Part model, mm, in its own coordinate system. Face numbers are marked on the shaded views. A direction names the side the tool comes from. Round coordinates to 2 decimals unless told otherwise and drop trailing zeros. Write each loop counter-clockwise with the first axis right and the second up, starting at its lowest first coordinate (ties: lowest second). Pieces come first, ordered by that corner, then holes. Notation, with made-up numbers: (44, 84) -> (87, 84) arc R16 cw to (87, 107) -> close; hole circle Ø8 at (67, -27.5). An arc over 180 degrees is marked (long way). Return JSON: item names as keys, results as strings. Group by question number.
(1) Saw through at C-C (y = 143). List the corners of the cut face in (x, z).
(2) Saw through at D-D (y = -368). List the corners of the cut face in (x, z).
(3) Drop flat-ended pins along their axis: pin 1 Ø6 at (y, z) = (-218, 209) entering from -X; pin 2 Ø4 at (x, z) = (337.5, 376.5) entering from -Y; pin 3 Ø6 at (x, y) = (418.5, -172) entering from +Z. Give the stop position or say it passes through.
(4) Drill centre lines: L1, parallel to Y at x = 434, z = 42.5; L2, parallel to Y at x = 382.5, z = 96; L3, parallel to Z at x = 487, y = 117.5. Where is each one in solid material? Low to high. Write a range as from..to.
(5) Mould opens along Z. For the marked faces 1, 2 and 3 say: +Z half, -Z half, draft (parallel to the pull), parting line (faces both ways), or undercut.
(6) Tool access for the marked faces 4, 5, 6 and 7: list every direction of +Z, -Z, +X, -X, +Y, -Y with a clear straight run to the whole face (end or side of a thin tool).
(7) Saw through at B-B (z = 155). State how many separate pieces and enclosed holes the cut face has, plus the area to 3 significant figures.
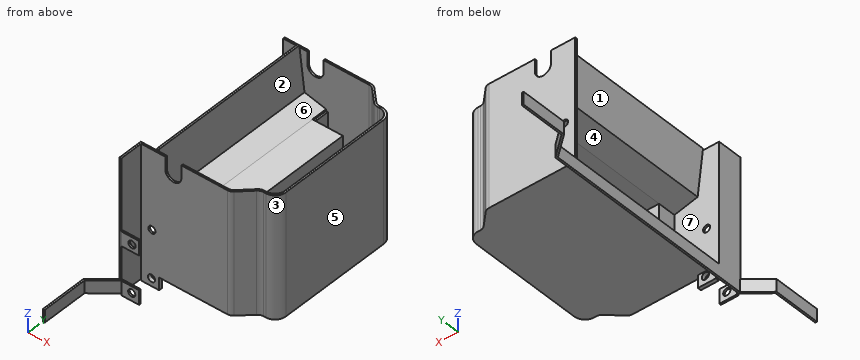
from build123d import *

# Parameters (mm, degrees)
F7_START  = 35
F7_DEPTH  = 5
F8_START  = 5
F8_DEPTH  = 35
F11_DEPTH = 200
F13_DEPTH = 369.76
F15_DEPTH = 45
F17_DEPTH = 45
F18_DEPTH = 45
F19_DEPTH = 45
F20_DEPTH = 335
F22_W     = 50.1510878829
F22_H     = 10
F23_DEPTH = 35
F24_W     = 5
F24_H     = 35
F24_H_2   = 5
F25_DEPTH = 50
F26_R     = 10
F27_DEPTH = 255.001
F29_DEPTH = 335
F30_W     = 5
F30_H     = 40
F31_DEPTH = 50
F32_R     = 10
F33_DEPTH = 780.001
F35_DEPTH = 715.001


with BuildPart() as f7:
    # F5 (on face) → F7 (new body)
    with BuildSketch(Plane.XY.offset(F7_START)):
        with BuildLine():
            Line((536.0502983732, 235), (295.2061215611, 235))
            Line((295.2061215611, 235), (295.2061215611, -235))
            Line((295.2061215611, -235), (536.0502983732, -235))
            ThreePointArc((536.0502983732, -235), (543.6023308733, -233.5193629782), (550.0361814825, -229.2966805117))
            Line((550.0361814825, -229.2966805117), (584.3760616397, -195.7033194883))
            ThreePointArc((584.3760616397, -195.7033194883), (590.8099122489, -191.4806370218), (598.361944749, -190))
            Line((598.361944749, -190), (605.2061215611, -190))
            ThreePointArc((605.2061215611, -190), (626.4193249967, -181.2132034356), (635.2061215611, -160))
            Line((635.2061215611, -160), (635.2061215611, 160))
            ThreePointArc((635.2061215611, 160), (626.4193249967, 181.2132034356), (605.2061215611, 190))
            Line((605.2061215611, 190), (598.361944749, 190))
            ThreePointArc((598.361944749, 190), (590.8099122489, 191.4806370218), (584.3760616397, 195.7033194883))
            Line((584.3760616397, 195.7033194883), (550.0361814825, 229.2966805117))
            ThreePointArc((550.0361814825, 229.2966805117), (543.6023308733, 233.5193629782), (536.0502983732, 235))
        make_face()
    extrude(amount=F7_DEPTH)

    # F10 (on face) → F11 (join)
    with BuildSketch(Plane.XY.offset(40)):
        Polygon((420.2061215611, 230), (415.2061215611, 230), (415.2061215611, 179.7606539726), (495.2061215611, 179.7606539726), (495.2061215611, -180), (415.2061215611, -180), (415.2061215611, -230), (420.2061215611, -230), (420.2061215611, -185), (500.2061215611, -185), (500.2061215611, 184.7606539726), (420.2061215611, 184.7606539726), align=None)
    extrude(amount=F11_DEPTH)



with BuildPart() as f8:
    # F6 (on face) → F8 (new body)
    with BuildSketch(Plane.XY.offset(F8_START)):
        Polygon((235.3396033727, 350), (235.3396033727, 480), (230.3396033727, 480), (230.3396033727, 347.6614641333), (290.2061215611, 297.6614641333), (290.2061215611, -297.6614641333), (230.3396033727, -347.6614641333), (230.3396033727, -480), (235.3396033727, -480), (235.3396033727, -350), (295.2061215611, -300), (295.2061215611, 300), align=None)
    extrude(amount=F8_DEPTH)


with BuildPart() as f13:
    # F12 (on face) → F13 (new body)
    with BuildSketch(Plane.XZ.offset(185)):
        Polygon((415.077149868, 240), (500.2061215611, 240), (500.2061215611, 245), (415.6496353582, 245), (354.7629135856, 259.1279170394), (340.264830222, 380.0120656257), (335.2289983824, 380.0120656257), (350.2161502838, 255.0500929356), align=None)
    extrude(amount=-F13_DEPTH)

    # F14 (on face) → F15 (join)
    with BuildSketch(Plane.XZ.offset(185)):
        Polygon((354.7629135856, 259.1279170394), (350.2161502838, 255.0500929356), (415.077149868, 240), (415.077149868, 245.1328372965), align=None)
    extrude(amount=F15_DEPTH)

    # F16 (on face) → F17 (join)
    with BuildSketch(Plane(origin=(0, 184.76, 0), x_dir=(-1, 0, 0), z_dir=(0, 1, 0))):
        Polygon((-415.077149868, 245.1328372965), (-415.077149868, 240), (-350.2161502838, 255.0500929356), (-354.7629135856, 259.1279170394), align=None)
    extrude(amount=F17_DEPTH)

    # F18 (add): a face of the model
    f18_faces = [f13.faces().sort_by_distance(p)[0] for p in [
        (345.1049776592, -185, 318.5448987695),
    ]]
    extrude(f18_faces, amount=F18_DEPTH)

    # F19 (add): a face of the model
    f19_faces = [f13.faces().sort_by_distance(p)[0] for p in [
        (345.1049776592, 184.76, 318.5448987695),
    ]]
    extrude(f19_faces, amount=F19_DEPTH)


with BuildPart() as f7_1:
    add(f7.part)

    add(f8.part)  # F20 merges F8

    add(f13.part)  # F20 merges F13
    # F9 (on face) → F20 (join)
    with BuildSketch(Plane.XY.offset(40)):
        with BuildLine():
            Line((536.0502983732, 235), (295.2061215611, 235))
            Line((295.2061215611, 235), (295.2061215611, 230))
            Line((295.2061215611, 230), (534.0113425762, 230))
            ThreePointArc((534.0113425762, 230), (541.5633750764, 228.5193629782), (547.9972256855, 224.2966805117))
            Line((547.9972256855, 224.2966805117), (582.3371058428, 190.7033194883))
            ThreePointArc((582.3371058428, 190.7033194883), (588.7709564519, 186.4806370218), (596.322988952, 185))
            Line((596.322988952, 185), (602.2061215611, 185))
            ThreePointArc((602.2061215611, 185), (622.0051114343, 176.7989898732), (630.2061215611, 157))
            Line((630.2061215611, 157), (630.2061215611, -157))
            ThreePointArc((630.2061215611, -157), (622.0051114343, -176.7989898732), (602.2061215611, -185))
            Line((602.2061215611, -185), (596.322988952, -185))
            ThreePointArc((596.322988952, -185), (588.7709564519, -186.4806370218), (582.3371058428, -190.7033194883))
            Line((582.3371058428, -190.7033194883), (547.9972256855, -224.2966805117))
            ThreePointArc((547.9972256855, -224.2966805117), (541.5633750764, -228.5193629782), (534.0113425762, -230))
            Line((534.0113425762, -230), (295.2061215611, -230))
            Line((295.2061215611, -230), (295.2061215611, -235))
            Line((295.2061215611, -235), (536.0502983732, -235))
            ThreePointArc((536.0502983732, -235), (543.6023308733, -233.5193629782), (550.0361814825, -229.2966805117))
            Line((550.0361814825, -229.2966805117), (584.3760616397, -195.7033194883))
            ThreePointArc((584.3760616397, -195.7033194883), (590.8099122489, -191.4806370218), (598.361944749, -190))
            Line((598.361944749, -190), (605.2061215611, -190))
            ThreePointArc((605.2061215611, -190), (626.4193249967, -181.2132034356), (635.2061215611, -160))
            Line((635.2061215611, -160), (635.2061215611, 160))
            ThreePointArc((635.2061215611, 160), (626.4193249967, 181.2132034356), (605.2061215611, 190))
            Line((605.2061215611, 190), (598.361944749, 190))
            ThreePointArc((598.361944749, 190), (590.8099122489, 191.4806370218), (584.3760616397, 195.7033194883))
            Line((584.3760616397, 195.7033194883), (550.0361814825, 229.2966805117))
            ThreePointArc((550.0361814825, 229.2966805117), (543.6023308733, 233.5193629782), (536.0502983732, 235))
        make_face()
    extrude(amount=F20_DEPTH)

    # F22 (on face) → F23 (join)
    with BuildSketch(Plane(origin=(0, 0, 35), x_dir=(1, 0, 0), z_dir=(0, 0, -1))):
        with Locations((320.2816655026, 230)):
            Rectangle(F22_W, F22_H)
    extrude(amount=F23_DEPTH)

    # F24 (on face) → F25 (join)
    with BuildSketch(Plane.YZ.offset(295.2061215611)):
        with Locations((-297.5, 22.5)):
            Rectangle(F24_W, F24_H)
        with Locations((-297.5, 2.5)):
            Rectangle(F24_W, F24_H_2)
    extrude(amount=F25_DEPTH)

    # F26 (on face) → F27 (cut, through all)
    with BuildSketch(Plane(origin=(0, -225, 0), x_dir=(-1, 0, 0), z_dir=(0, 1, 0))):
        with Locations((-324.3654668331, 21.796002984)):
            Circle(F26_R)
    extrude(amount=-F27_DEPTH, mode=Mode.SUBTRACT)

    # F28 (on face) → F29 (join)
    with BuildSketch(Plane.XY.offset(40)):
        Polygon((295.2061215611, -235), (295.2061215611, -230), (290.2061215611, -230), (290.2061215611, -297.6614641333), (290.2061215611, -300.0012075878), (295.2046756796, -300.0012075878), (295.2061215611, -300), (295.2061215611, -295), align=None)
    extrude(amount=F29_DEPTH)

    # F30 (on face) → F31 (join)
    with BuildSketch(Plane.YZ.offset(295.2061215611)):
        with Locations((-297.5, 155)):
            Rectangle(F30_W, F30_H)
    extrude(amount=F31_DEPTH)

    # F32 (on face) → F33 (cut, through all)
    with BuildSketch(Plane.XZ.offset(300)):
        with Locations((325.2061215611, 155)):
            Circle(F32_R)
    extrude(amount=-F33_DEPTH, mode=Mode.SUBTRACT)

    # F34 (on face) → F35 (cut, through all)
    with BuildSketch(Plane.XZ.offset(235)):
        with BuildLine():
            Line((362.7061215611, 375), (362.7061215611, 340))
            ThreePointArc((362.7061215611, 340), (385.2061215611, 317.5), (407.7061215611, 340))
            Line((407.7061215611, 340), (407.7061215611, 375))
            Line((407.7061215611, 375), (362.7061215611, 375))
        make_face()
    extrude(amount=-F35_DEPTH, mode=Mode.SUBTRACT)


solid = f7_1.part
Computed values:
{
 "1": {"outline": "(290.21, 5) -> (295.21, 5) -> (295.21, 35) -> (635.21, 35) -> (635.21, 375) -> (630.21, 375) -> (630.21, 40) -> (500.21, 40) -> (500.21, 245) -> (415.65, 245) -> (354.76, 259.13) -> (340.26, 380.01) -> (335.23, 380.01) -> (350.22, 255.05) -> (415.08, 240) -> (495.21, 240) -> (495.21, 40) -> (290.21, 40) -> close"},
 "2": {"outline": "(230.34, 5) -> (235.34, 5) -> (235.34, 40) -> (230.34, 40) -> close"},
 "3": {"pin 1": "x = 415.21", "pin 2": "y = -235", "pin 3": "z = 245.03"},
 "4": {"L1": "-235..-230, -185..-180, 179.76..184.76, 230..235", "L2": "-235..-230, 230..235", "L3": "35..40, 240..245"},
 "5": {"face 1": "undercut", "face 2": "+Z half", "face 3": "draft"},
 "6": {"face 4": "-X", "face 5": "+Z, -Z, +X, +Y, -Y", "face 6": "+Z", "face 7": "none"},
 "7": {"separate pieces": "4", "enclosed holes": "1", "area": "8,780 mm2"}
}
